```python
from build123d import *

# Parameters (mm, degrees)
ESQUISSE1_W           = 10
ESQUISSE1_H           = 20
EXTRUSION1_DEPTH      = 20
EXTRUSION2_DEPTH      = 23.912878475
EXTRUSION2_DEPTH_BACK = 23.912878475
ESQUISSE4_R           = 1.5
EXTRUSION3_DEPTH      = 40


with BuildPart() as part:
    # Esquisse1 → Extrusion1 (new body)
    with BuildSketch(Plane.XY):
        Rectangle(ESQUISSE1_W, ESQUISSE1_H)
    extrude(amount=EXTRUSION1_DEPTH)

    # Esquisse3 → Extrusion2 (cut, two sides: drawn at the far end of the back side and taken through both)
    with BuildSketch(Plane.XY.offset(20).offset(-EXTRUSION2_DEPTH_BACK)):
        Polygon((-38.75439594, 39.75439594), (-5, 6), (-2.5, 3.5), (-5, 1), (-38.75439594, -32.75439594), (-134.226244997, -32.75439594), (-134.226244997, 39.75439594), align=None)
    extrude(amount=EXTRUSION2_DEPTH + EXTRUSION2_DEPTH_BACK, mode=Mode.SUBTRACT)

    # Esquisse4 → Extrusion3 (cut)
    with BuildSketch(Plane(origin=(5, 0, 0), x_dir=(0, 0, -1), z_dir=(1, 0, 0))):
        with Locations((-10, -5)):
            Circle(ESQUISSE4_R)
    extrude(amount=-EXTRUSION3_DEPTH, mode=Mode.SUBTRACT)


solid = part.part
```
For this review, take the finished solid that the model builds, in its own axes (mm). A direction names the side the tool comes from. Round coordinates to 2 decimals unless told otherwise and drop trailing zeros. Write each loop counter-clockwise with the first axis right and the second up, starting at its lowest first coordinate (ties: lowest second). Pieces come first, ordered by that corner, then holes. Notation, with made-up numbers: (59.5, 18.5) -> (100.5, 18.5) arc R25 ccw to (100.5, 30.5) -> close; hole circle Ø11 at (84, 75.25). An arc over 180 degrees is marked (long way). One line per question, with ' | ' between items. Start each with the question number.
(1) Insertion check: P1, Ø2.5, axis at y = -5, z = 10, coming from the +X side. The pin has a flat end and moves straight along its axis. Give the tip position at first contact, or say it passes through.
(2) Add section B-B, the plane y = -5. Write out the cut boundary in (x, z).
(3) For line 1 along Y through (x, z) = (-0.75, 10); line 2 along Y through (x, z) = (-3.25, 9.5); line 3 along X through (y, z) = (2.5, 4.5), list the stretches that pass through material, from the lowest coordinate up. Write a range as from..to.
(4) Add section C-C, the plane z = 10. Write out the cut boundary in (x, y), plus the area to 3 significant figures.
(5) Add section D-D, the plane z = 12.75. Write out the cut boundary in (x, y), plus the area to 3 significant figures.
(6) Add section A-A, the plane x = -3.5. Write out the cut boundary in (y, z), plus the area to 3 significant figures.
(7) Tool access review of faces 1 (the face through (-4, 2, 10)), 2 (the face through (0, 10, 10)): name each direction out of +Z, -Z, +X, -X, +Y, -Y from which nothing blocks a thin tool from reaching the whole face with its end or side.
(8) Mouldability with a two-part tool opening along Y and no side actions: class faces 3 (the face through (5, 0, 10)), 4 (the face through (0, -10, 10)), 5 (the face through (-4, 5, 10)) as released by +Y, released by -Y, zero draft, split by the parting line, or undercut.
Answer list:
1) P1: through
2) outline: (-5, 0) -> (5, 0) -> (5, 8.5) -> (-5, 8.5) -> close; (-5, 11.5) -> (5, 11.5) -> (5, 20) -> (-5, 20) -> close
3) line 1: -10..-6.5, -3.5..10 | line 2: -10..-6.41, -3.59..2.75, 4.25..10 | line 3: -3.5..5
4) outline: (-5, -10) -> (5, -10) -> (5, -6.5) -> (-5, -6.5) -> close; (-5, -3.5) -> (5, -3.5) -> (5, 10) -> (-5, 10) -> (-5, 6) -> (-2.5, 3.5) -> (-5, 1) -> close | area: 164 mm²
5) outline: (-5, -10) -> (5, -10) -> (5, 10) -> (-5, 10) -> (-5, 6) -> (-2.5, 3.5) -> (-5, 1) -> close | area: 194 mm²
6) outline: (-10, 0) -> (2.5, 0) -> (2.5, 20) -> (-10, 20) -> close; (4.5, 0) -> (10, 0) -> (10, 20) -> (4.5, 20) -> close; hole circle Ø3 at (-5, 10) | area: 353 mm²
7) face 1: +Z, -Z, -X | face 2: +Z, -Z, +X, -X, +Y
8) face 3: zero draft | face 4: released by -Y | face 5: undercut
